CAD build for the part. Positions are in the model's coordinates, mm. A direction names the side the tool comes from. Give positions to 0.01 mm unless a question says otherwise; leave off trailing zeros. Write each loop counter-clockwise with the first axis right and the second up, starting at its lowest first coordinate (ties: lowest second). Pieces come first, ordered by that corner, then holes. Notation, with made-up numbers: M 3,-25 L 37,-25 A27 ccw 37,11 Z; hole C -9.5,-31.5 d11. An arc over 180 degrees is marked long. One line per question, with ' | ' between items. Start each with the question number.
1. Cut at D-D, the plane y = 4.25. Write the cut outline in (x, z) (3 decimals).
2. Flat gauge pins, fed straight in: pin 1 (5 mm diameter, centred on x = 2, y = 14, fed in from +Z); pin 2 (3 mm diameter, centred on x = 4, y = -4, fed in from +Z); pin 3 (1.6 mm diameter, centred on x = 5.5, z = -46.5, fed in from +Y). Where does each tip first touch, or does it go through?
3. Cut at A-A, the plane y = -3.25. Write the cut outline in (x, z), then the cut area to 3 significant figures.
4. Which spindle directions (+Z, -Z, +X, -X, +Y, -Y) get a long thin tool onto all of the face, cutting with end or side? Do faces 1 (the face through (7.938, -3, -6)), 2 (the face through (5, -3, -3.217)), 3 (the face through (6.35, 6.7, -38.3)), 4 (the face through (5, 7, -36.078)). Say none if no direction does.
5. Pull direction Z, two halves, no side cores. Call faces 5 (the face through (5, 2, 0)), 6 (the face through (5, 7, -12.785)), 7 (the face through (7.938, -3, -43)): released by +Z, released by -Z, zero draft, split by the parting line, or undercut.
6. Wall check: L1, parallel to Z at x = 3.75, y = 0.75; L2, parallel to Z at x = 6, y = 7; L3, parallel to Z at x = 1, y = 6.5. Give the ranges that are in metal, low to high.
```python
from build123d import *

# Parameters (mm, degrees)
BOSS_EXTRUDE1_DEPTH = 9.525
SKETCH3_R           = 0.508
CUT_EXTRUDE2_DEPTH  = 6.35
FILLET1_R           = 1.5875
ESQUISSE1_W         = 6.35
ESQUISSE1_H         = 6.35
BOSS_EXTRU_1_DEPTH  = 6.35


with BuildPart() as part:
    # Sketch1 → Boss-Extrude1 (new body)
    with BuildSketch(Plane(origin=(0, 0, 0), x_dir=(0, 0, -1), z_dir=(1, 0, 0))):
        Polygon((0, 0), (12.7847852, 0), (12.7847852, 13.390245), (36.0778552, 13.390245), (36.0778552, 0), (48.8626404, 0), (48.8626404, 4.7625), (42.4278552, 4.7625), (42.4278552, 19.740245), (41.4309052, 19.740245), (6.3509652, 19.740245), (6.3509652, 4.7625), (0, 4.7625), align=None)
    extrude(amount=BOSS_EXTRUDE1_DEPTH)

    # Sketch3 → Cut-Extrude2 (cut)
    with BuildSketch(Plane.ZY):
        with Locations((-38.3232152, 6.68528)):
            Circle(SKETCH3_R)
        with Locations((-10.5229152, 6.6951225)):
            Circle(SKETCH3_R)
    extrude(amount=-CUT_EXTRUDE2_DEPTH, mode=Mode.SUBTRACT)

    # Fillet1
    fillet1_edges = [part.edges().sort_by_distance(p)[0] for p in [
        (4.7625, 4.7625, 0),
        (4.7625, 4.7625, -6.3509652),
        (4.7625, 19.740245, -6.3509652),
        (4.7625, 19.740245, -42.4278552),
        (4.7625, 4.7625, -42.4278552),
        (4.7625, 4.7625, -48.8626404),
    ]]
    fillet(fillet1_edges, radius=FILLET1_R)

    # Esquisse1 → Boss.-Extru.1 (add)
    with BuildSketch(Plane.XZ):
        with Locations((4.7625, -42.4702478)):
            Rectangle(ESQUISSE1_W, ESQUISSE1_H)
        with Locations((4.7625, -6.3923926)):
            Rectangle(ESQUISSE1_W, ESQUISSE1_H)
    extrude(amount=BOSS_EXTRU_1_DEPTH)


solid = part.part
```
Here are the results:
1) outline: M 0,-48.443 L 9.525,-48.443 L 9.525,-36.078 L 0,-36.078 Z; M 0,-12.785 L 9.525,-12.785 L 9.525,-0.419 L 0,-0.419 Z
2) pin 1: z = -6.35 | pin 2: z = -3.22 | pin 3: y = 4.76
3) outline: M 1.59,-45.65 L 7.94,-45.65 L 7.94,-39.3 L 1.59,-39.3 Z; M 1.59,-9.57 L 7.94,-9.57 L 7.94,-3.22 L 1.59,-3.22 Z | area: 80.6 mm^2
4) face 1: +Z, -Z, +X, -Y | face 2: +Z, +X, -X, -Y | face 3: -X | face 4: +X, -X, -Y
5) face 5: released by +Z | face 6: undercut | face 7: zero draft
6) L1: -48.86 to -36.08, -12.78 to 0 | L2: -42.43 to -38.72, -37.92 to -36.08, -12.78 to -10.93, -10.12 to -6.35 | L3: -42.43 to -38.8, -37.85 to -36.08, -12.78 to -10.99, -10.05 to -6.35
